Read the model definition and answer for the solid it produces. Units are mm, in the model's axes. Face numbers are marked on the shaded views. A direction names the side the tool comes from. Give positions to 0.01 mm unless a question says otherwise; leave off trailing zeros. Order: outer loops, then holes, each group sorted by start corner. A loop starts at its lowest first (then second) coordinate and runs counter-clockwise, first axis right, second up. Notation, with made-up numbers: M -1.75,85 L 7.25,85 A19 cw 7.25,107 Z; hole C 1.25,-17.5 d3. An arc over 180 degrees is marked long. One line per item, written item: value.
from build123d import *

# Parameters (mm, degrees)
SKETCH1_W           = 25.4
SKETCH1_H           = 50.8
BOSS_EXTRUDE1_DEPTH = 61.9125
SHELL1_T            = -3.175


with BuildPart() as part:
    # Sketch1 → Boss-Extrude1 (new body, symmetric)
    with BuildSketch(Plane.XY):
        Rectangle(SKETCH1_W, SKETCH1_H)
    extrude(amount=BOSS_EXTRUDE1_DEPTH, both=True)

    # Shell1
    shell1_openings = [part.faces().sort_by_distance(p)[0] for p in [
        (0, 0, 61.9125),
        (0, 0, -61.9125),
    ]]
    offset(amount=SHELL1_T, openings=shell1_openings, kind=Kind.INTERSECTION)


solid = part.part
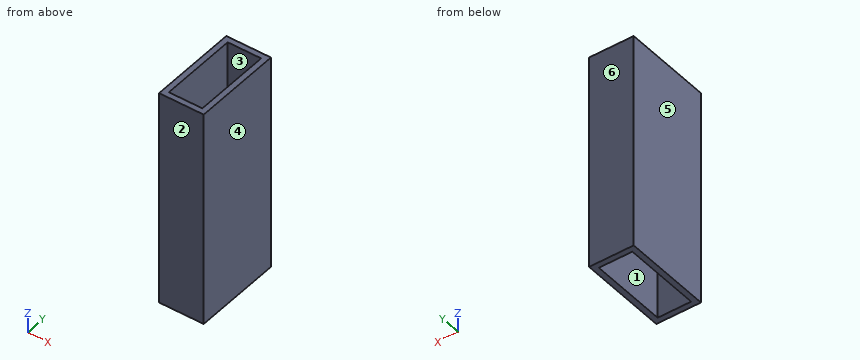
1) Find section C-C, the plane y = 20. Write down the section's boundary in (x, z) (1 decimal), plus the area to 3 significant figures.
Reported:
outline: M -12.7,-61.9 L -9.5,-61.9 L -9.5,61.9 L -12.7,61.9 Z; M 9.5,-61.9 L 12.7,-61.9 L 12.7,61.9 L 9.5,61.9 Z
area: 786 mm^2
2) Find section A-A, the plane x = 6.5. Write down the section's boundary in (y, z) (1 decimal), plus the area to 3 significant figures.
Reported:
outline: M -25.4,-61.9 L -22.2,-61.9 L -22.2,61.9 L -25.4,61.9 Z; M 22.2,-61.9 L 25.4,-61.9 L 25.4,61.9 L 22.2,61.9 Z
area: 786 mm^2
3) Determine the mould class of the marked faces 3, 4, 5 and 6 for opening direction X: +X half, -X half, draft (parallel to the pull), parting line (faces both ways), or undercut.
Reported:
face 3: undercut
face 4: +X half
face 5: -X half
face 6: draft
4) Consider probe 1 along X at (y, z) = (-6.5, 3) (3 decimals); probe 2 along Y at (x, z) = (-5.75, 37.5) (3 decimals). Determine where each line is inside the solid, lowest interval first.
Reported:
probe 1: x = -12.7 to -9.525, 9.525 to 12.7
probe 2: y = -25.4 to -22.225, 22.225 to 25.4
5) Find section B-B, the plane z = -7. Write down the section's boundary in (x, y) (3 decimals).
Reported:
outline: M -12.7,-25.4 L 12.7,-25.4 L 12.7,25.4 L -12.7,25.4 Z; hole M -9.525,-22.225 L 9.525,-22.225 L 9.525,22.225 L -9.525,22.225 Z
6) Which of the six approach directions +Z, -Z, +X, -X, +Y, -Y give full straight-line access (tool end or side, diameter ignored) to the marked faces 1 and 2?
Reported:
face 1: +Z, -Z
face 2: +Z, -Z, +X, -X, -Y
